Job drawing, mm, ordinate dimensions from the low corner. One solid piece. Give positions to 0.01 mm unless a question says otherwise; leave off trailing zeros. Loops run counter-clockwise (first coordinate to the right, second up) from the corner with the lowest first, then second, coordinate; pieces in that order, holes last. Notation, with made-up numbers: (54.25, 33.5) -> (107.25, 33.5) arc R25 ccw to (107.25, 72.5) -> close; hole circle Ø2 at (58, 16). An arc over 180 degrees is marked (long way). Use one line per item in the form item = value.
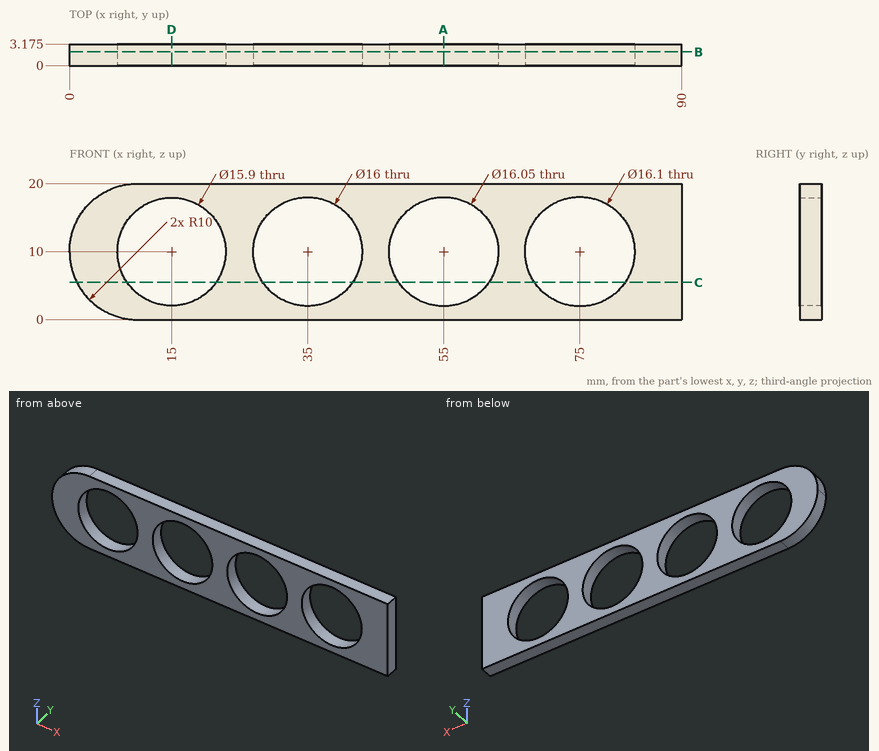
1. Cut at C-C, the plane z = 5.5. Write the cut outline in (x, y) (1 decimal), then the cut area to 3 significant figures.
Result sheet:
outline = (1.1, 0) -> (8.4, 0) -> (8.4, 3.2) -> (1.1, 3.2) -> close; (21.6, 0) -> (28.4, 0) -> (28.4, 3.2) -> (21.6, 3.2) -> close; (41.6, 0) -> (48.4, 0) -> (48.4, 3.2) -> (41.6, 3.2) -> close; (61.6, 0) -> (68.3, 0) -> (68.3, 3.2) -> (61.6, 3.2) -> close; (81.7, 0) -> (90, 0) -> (90, 3.2) -> (81.7, 3.2) -> close
area = 114 mm^2
2. Cut at A-A, the plane x = 55. Write the cut outline in (y, z) (3 decimals), then the cut area to 3 significant figures.
Result sheet:
outline = (0, 0) -> (3.175, 0) -> (3.175, 1.975) -> (0, 1.975) -> close; (0, 18.025) -> (3.175, 18.025) -> (3.175, 20) -> (0, 20) -> close
area = 12.5 mm^2
3. Cut at D-D, the plane x = 15. Write the cut outline in (y, z) (3 decimals), then the cut area to 3 significant figures.
Result sheet:
outline = (0, 0) -> (3.175, 0) -> (3.175, 2.05) -> (0, 2.05) -> close; (0, 17.95) -> (3.175, 17.95) -> (3.175, 20) -> (0, 20) -> close
area = 13.0 mm^2
4. Cut at B-B, the plane y = 2. State how many separate pieces and enclosed holes the cut face has.
Result sheet:
separate_pieces = 1
enclosed_holes = 4
5. Drill centre lines: line 1 (X direction, y = 2.25, z = 10) (3 decimals); line 2 (X direction, y = 1.35, z = 12.5); line 3 (Z direction, x = 74.5, y = 2.75). Where is each one in solid material? Low to high.
Result sheet:
line_1 = 0 to 7.05, 22.95 to 27, 43 to 46.975, 63.025 to 66.95, 83.05 to 90
line_2 = 0.32 to 7.45, 22.55 to 27.4, 42.6 to 47.37, 62.63 to 67.35, 82.65 to 90
line_3 = 0 to 1.97, 18.03 to 20
